```python
from build123d import *

# Parameters (mm, degrees)
SKETCH1_R               = 2.1
SKETCH1_R_2             = 3.4
PROFILE_LENGTH_DEPTH    = 30
CUT_EXTRUDE1_DEPTH      = 37.742346142
CUT_EXTRUDE1_DEPTH_BACK = 37.742346142
SKETCH2_R               = 5


with BuildPart() as part:
    # Sketch1 → profile length (new, symmetric)
    with BuildSketch(Plane(origin=(0, 0, 0), x_dir=(1, 0, 0), z_dir=(0, 1, 0))):
        with BuildLine():
            Line((-4, 15), (-4, 13))
            Line((-4, 13), (-8.25, 13))
            Line((-8.25, 13), (-8.25, 9.664213562))
            Line((-8.25, 9.664213562), (-4.585786438, 6))
            Line((-4.585786438, 6), (4.585786438, 6))
            Line((4.585786438, 6), (8.25, 9.664213562))
            Line((8.25, 9.664213562), (8.25, 13))
            Line((8.25, 13), (4, 13))
            Line((4, 13), (4, 15))
            Line((4, 15), (13, 15))
            ThreePointArc((13, 15), (14.414213562, 14.414213562), (15, 13))
            Line((15, 13), (15, 4))
            Line((15, 4), (13, 4))
            Line((13, 4), (13, 8.25))
            Line((13, 8.25), (9.664213562, 8.25))
            Line((9.664213562, 8.25), (6, 4.585786438))
            Line((6, 4.585786438), (6, -4.585786438))
            Line((6, -4.585786438), (9.664213562, -8.25))
            Line((9.664213562, -8.25), (13, -8.25))
            Line((13, -8.25), (13, -4))
            Line((13, -4), (15, -4))
            Line((15, -4), (15, -13))
            ThreePointArc((15, -13), (14.414213562, -14.414213562), (13, -15))
            Line((13, -15), (4, -15))
            Line((4, -15), (4, -13))
            Line((4, -13), (8.25, -13))
            Line((8.25, -13), (8.25, -9.664213562))
            Line((8.25, -9.664213562), (4.585786438, -6))
            Line((4.585786438, -6), (-4.585786438, -6))
            Line((-4.585786438, -6), (-8.25, -9.664213562))
            Line((-8.25, -9.664213562), (-8.25, -13))
            Line((-8.25, -13), (-4, -13))
            Line((-4, -13), (-4, -15))
            Line((-4, -15), (-13, -15))
            ThreePointArc((-13, -15), (-14.414213562, -14.414213562), (-15, -13))
            Line((-15, -13), (-15, -4))
            Line((-15, -4), (-13, -4))
            Line((-13, -4), (-13, -8.25))
            Line((-13, -8.25), (-9.664213562, -8.25))
            Line((-9.664213562, -8.25), (-6, -4.585786438))
            Line((-6, -4.585786438), (-6, 4.585786438))
            Line((-6, 4.585786438), (-9.664213562, 8.25))
            Line((-9.664213562, 8.25), (-13, 8.25))
            Line((-13, 8.25), (-13, 4))
            Line((-13, 4), (-15, 4))
            Line((-15, 4), (-15, 13))
            ThreePointArc((-15, 13), (-14.414213562, 14.414213562), (-13, 15))
            Line((-13, 15), (-4, 15))
        make_face()
        with Locations(Location((-11.6, 11.6, 0), (0, 0, 270))):
            Circle(SKETCH1_R, mode=Mode.SUBTRACT)
        with Locations(Location((11.6, 11.6, 0), (0, 0, 90))):
            Circle(SKETCH1_R, mode=Mode.SUBTRACT)
        with Locations(Location((11.6, -11.6, 0), (0, 0, 270))):
            Circle(SKETCH1_R, mode=Mode.SUBTRACT)
        with Locations(Location((-11.6, -11.6, 0), (0, 0, 90))):
            Circle(SKETCH1_R, mode=Mode.SUBTRACT)
        with Locations(Location((0, 0, 0), (0, 0, 270))):
            Circle(SKETCH1_R_2, mode=Mode.SUBTRACT)
    extrude(amount=PROFILE_LENGTH_DEPTH, both=True)

    # Sketch2 → Cut-Extrude1 (cut, two sides: drawn at the far end of the back side and taken through both)
    with BuildSketch(Plane(origin=(0, 0, 0), x_dir=(0, 0, -1), z_dir=(1, 0, 0)).offset(-CUT_EXTRUDE1_DEPTH_BACK)):
        with Locations(Location((0, -15, 0), (0, 0, 23.486027641))):
            Circle(SKETCH2_R)
    extrude(amount=CUT_EXTRUDE1_DEPTH + CUT_EXTRUDE1_DEPTH_BACK, mode=Mode.SUBTRACT)


solid = part.part
```
Work out the finished part from the listing and answer in its coordinate system (mm). A direction names the side the tool comes from. Give positions to 0.01 mm unless a question says otherwise; leave off trailing zeros. Loops run counter-clockwise (first coordinate to the right, second up) from the corner with the lowest first, then second, coordinate; pieces in that order, holes last. Notation, with made-up numbers: M 61,35.25 L 103,35.25 A28 cw 103,58.25 Z; hole C 31,40 d9. An arc over 180 degrees is marked long. One line per item, written item: value. Start each with the question number.
1. Find section D-D (y = -15). State how many separate pieces and enclosed holes the cut face has, and give its area (3 significant figures).
2. Find section B-B (z = 11.6). Give the vertices of the cut face in (x, y), and give its area (3 significant figures).
3. Find the intervals of material crossed by probe 1 along Z at (x, y) = (-4.25, -21); probe 2 along X at (y, z) = (0.5, -11.6); probe 3 along Z at (x, y) = (0, -25.75), in increasing order.
4. Which of the six approach directions +Z, -Z, +X, -X, +Y, -Y give full straight-line access (tool end or side, diameter ignored) to faces 1 (the face through (-14, -15, 5)), 2 (the face through (-6, -25, 0)), 3 (the face through (14, 9, -4))?
5. Find section A-A (x = -11.6). Give the vertices of the cut face in (y, z).
6. Each of these flat-tipped pins is pushed along its axis until it touches: P1, Ø0.6, axis at x = -14, y = 17, coming from the -Z side; P2, Ø1, axis at x = -14, y = 3.5, coming from the +Z side. Where does it stop, or does it pass through?
7. Find section C-C (x = 0). Give the vertices of the cut face in (y, z), and give its area (3 significant figures).
8. Determine the mould class of faces 4 (the face through (15, 0, -9)), 5 (the face through (14, 9, 4)), 6 (the face through (13, 0, 6)) for opening direction X: released by +X, released by -X, zero draft, split by the parting line, or undercut.
Reported:
1. separate pieces: 2
1. enclosed holes: 4
1. area: 241 mm²
2. outline: M -15,-30 L -13.7,-30 L -13.7,30 L -15,30 Z; M -9.5,-30 L -8.25,-30 L -8.25,30 L -9.5,30 Z; M 8.25,-30 L 9.5,-30 L 9.5,30 L 8.25,30 Z; M 13.7,-30 L 15,-30 L 15,30 L 13.7,30 Z
2. area: 306 mm²
3. probe 1: z = -15 to -13, -6 to 6, 13 to 15
3. probe 2: x = -15 to -13.7, -9.5 to -8.25, 8.25 to 9.5, 13.7 to 15
3. probe 3: z = -6 to -3.4, 3.4 to 6
4. face 1: +X, -X
4. face 2: +Y, -Y
4. face 3: +X, +Y, -Y
5. outline: M -30,-15 L 30,-15 L 30,-13.7 L -30,-13.7 Z; M -30,-9.5 L 30,-9.5 L 30,-8.25 L -30,-8.25 Z; M -30,8.25 L 30,8.25 L 30,9.5 L -30,9.5 Z; M -30,13.7 L 30,13.7 L 30,15 L -30,15 Z
6. P1: stops at z = -14.87
6. P2: stops at z = 14.94
7. outline: M -30,-6 L 30,-6 L 30,-3.4 L -11.33,-3.4 A5 cw -18.67,-3.4 L -30,-3.4 Z; M -30,3.4 L -18.67,3.4 A5 cw -11.33,3.4 L 30,3.4 L 30,6 L -30,6 Z
7. area: 296 mm²
8. face 4: released by +X
8. face 5: zero draft
8. face 6: undercut
